Autodesk Inventor part; units mm, degrees
ref_plane "at507h_XY" through (0, 16.3576, 0) normal (0, 1, 0) x (1, 0, 0)
ref_plane "at507h_YZ" through (0, 16.3576, 0) normal (1, 0, 0) x (0, 0, -1)
ref_plane "at507h_ZX" through (0, 16.3576, 0) normal (0, 0, -1) x (0, 1, 0)
sketch "Sketch_1" plane through (0, 0, 0) normal (1, 0, 0) x (0, 1, 0)
  line L0 (12.8016, 6.5024) -> (9.7536, 6.5024)
  line L1 (9.7536, 6.5024) -> (9.7536, 5.4864)
  arc A0 (9.2456, 4.9784) -> (9.7536, 5.4864) centre (9.2456, 5.4864) ccw
  line L2 (9.2456, 4.9784) -> (2.54, 4.9784)
  line L3 (2.54, 4.9784) -> (2.54, -4.9784)
  line L4 (2.54, -4.9784) -> (9.2456, -4.9784)
  arc A1 (9.7536, -5.4864) -> (9.2456, -4.9784) centre (9.2456, -5.4864) ccw
  line L5 (9.7536, -5.4864) -> (9.7536, -6.5024)
  line L6 (9.7536, -6.5024) -> (12.8016, -6.5024)
  arc A2 (12.8016, -6.5024) -> (13.0556, -6.2484) centre (12.8016, -6.2484) ccw
  line L7 (13.0556, -6.2484) -> (13.0556, 6.2484)
  arc A3 (13.0556, 6.2484) -> (12.8016, 6.5024) centre (12.8016, 6.2484) ccw
extrude "Extrusion1" add sketch "Sketch_1" along normal mid plane 12.7
sketch "Sketch_2" plane through (0, 0, 0) normal (0, 1, 0) x (-1, 0, 0)
  line L0 (6.096, 6.2484) -> (-6.096, 6.2484)
  line L1 (-6.096, 6.2484) -> (-6.096, -6.2484)
  line L2 (-6.096, -6.2484) -> (6.096, -6.2484)
  line L3 (6.096, -6.2484) -> (6.096, 6.2484)
extrude "Extrusion2" cut sketch "Sketch_2" along normal blind 12.8016
sketch "Sketch_3" plane through (0, 0, 0) normal (0, 0, 1) x (1, 0, 0)
  line L0 (-6.35, 15.24) -> (-6.35, 12.8016)
  arc A0 (-6.096, 13.0556) -> (-6.35, 12.8016) centre (-6.096, 12.8016) ccw
  line L1 (-6.096, 13.0556) -> (6.096, 13.0556)
  arc A1 (6.35, 12.8016) -> (6.096, 13.0556) centre (6.096, 12.8016) ccw
  line L2 (6.35, 12.8016) -> (6.35, 15.24)
  line L3 (6.35, 15.24) -> (-6.35, 15.24)
extrude "Extrusion3" cut sketch "Sketch_3" along normal mid plane 25.6032
sketch "Sketch_4" plane through (0, 2.54, 0) normal (0, 1, 0) x (1, 0, 0)
  line L0 (-6.096, 5.4864) -> (-6.096, -5.4864)
  line L1 (-6.096, -5.4864) -> (-6.35, -5.4864)
  line L2 (-6.35, -5.4864) -> (-6.35, 5.4864)
  line L3 (-6.35, 5.4864) -> (-6.096, 5.4864)
  line L4 (-6.096, 5.4864) -> (-6.096, -5.4864)
revolve "Revolution1" add sketch "Sketch_4" angle 90 about axis through (-6.096, 2.54, -5.4864) along (0, 0, 1)
sketch "Sketch_5" plane through (0, 2.54, 0) normal (0, 1, 0) x (1, 0, 0)
  line L0 (6.096, -5.4864) -> (6.096, 5.4864)
  line L1 (6.096, 5.4864) -> (6.35, 5.4864)
  line L2 (6.35, 5.4864) -> (6.35, -5.4864)
  line L3 (6.35, -5.4864) -> (6.096, -5.4864)
  line L4 (6.096, -5.4864) -> (6.096, 5.4864)
revolve "Revolution2" add sketch "Sketch_5" angle 90 about axis through (6.096, 2.54, 5.4864) along (0, 0, -1)
sketch "Sketch_6" plane through (0, 2.54, 0) normal (0, 1, 0) x (1, 0, 0)
  line L0 (-6.096, 2.7305) -> (-6.096, -2.7305)
  line L1 (-6.096, -2.7305) -> (-5.715, -2.7305)
  arc A0 (-5.715, -2.7305) -> (-5.715, -1.9685) centre (-5.715, -2.3495) ccw
  line L2 (-5.715, -1.9685) -> (-5.715, 1.9685)
  arc A1 (-5.715, 1.9685) -> (-5.715, 2.7305) centre (-5.715, 2.3495) ccw
  line L3 (-5.715, 2.7305) -> (-6.096, 2.7305)
extrude "Extrusion4" add sketch "Sketch_6" against normal blind 0.254
sketch "Sketch_7" plane through (0, 2.54, 0) normal (0, 1, 0) x (1, 0, 0)
  arc A0 (5.715, 2.7305) -> (5.715, 1.9685) centre (5.715, 2.3495) ccw
  line L0 (5.715, 1.9685) -> (5.715, -1.9685)
  arc A1 (5.715, -1.9685) -> (5.715, -2.7305) centre (5.715, -2.3495) ccw
  line L1 (5.715, -2.7305) -> (6.096, -2.7305)
  line L2 (6.096, -2.7305) -> (6.096, 2.7305)
  line L3 (6.096, 2.7305) -> (5.715, 2.7305)
extrude "Extrusion5" add sketch "Sketch_7" against normal blind 0.254
sketch "Sketch_8" plane through (6.35, 0, 0) normal (1, 0, 0) x (0, 0, -1)
  line L0 (-7.1863, 0) -> (7.752, 0)
  line L1 (7.752, 0) -> (7.752, 3.302)
  line L2 (7.752, 3.302) -> (4.9784, 3.302)
  arc A0 (4.7244, 3.048) -> (4.9784, 3.302) centre (4.7244, 3.302) ccw
  line L3 (4.7244, 3.048) -> (2.9845, 3.048)
  arc A1 (2.9845, 3.048) -> (2.7305, 2.794) centre (2.9845, 2.794) ccw
  line L4 (2.7305, 2.794) -> (2.7305, 2.286)
  line L5 (2.7305, 2.286) -> (1.9685, 2.286)
  line L6 (1.9685, 2.286) -> (1.9685, 2.794)
  arc A2 (1.9685, 2.794) -> (1.7145, 3.048) centre (1.7145, 2.794) ccw
  line L7 (1.7145, 3.048) -> (-1.7145, 3.048)
  arc A3 (-1.7145, 3.048) -> (-1.9685, 2.794) centre (-1.7145, 2.794) ccw
  line L8 (-1.9685, 2.794) -> (-1.9685, 2.286)
  line L9 (-1.9685, 2.286) -> (-2.7305, 2.286)
  line L10 (-2.7305, 2.286) -> (-2.7305, 2.794)
  arc A4 (-2.7305, 2.794) -> (-2.9845, 3.048) centre (-2.9845, 2.794) ccw
  line L11 (-2.9845, 3.048) -> (-4.7244, 3.048)
  arc A5 (-4.9784, 3.302) -> (-4.7244, 3.048) centre (-4.7244, 3.302) ccw
  line L12 (-4.9784, 3.302) -> (-7.1863, 3.302)
  line L13 (-7.1863, 3.302) -> (-7.1863, 0)
extrude "Extrusion6" cut sketch "Sketch_8" against normal blind 25.4
sketch "Sketch_17" plane through (0, 0, 0) normal (0, 0, 1) x (1, 0, 0)
  line L0 (0, 13.0556) -> (0, 21.9456)
  line L1 (0, 21.9456) -> (3.175, 21.9456)
  line L2 (3.175, 21.9456) -> (3.175, 13.9446)
  line L3 (3.175, 13.9446) -> (3.683, 13.9446)
  line L4 (3.683, 13.9446) -> (3.683, 13.0556)
  line L5 (3.683, 13.0556) -> (0, 13.0556)
  line L6 (0, 13.0556) -> (0, 21.9456)
revolve "Revolution3" add sketch "Sketch_17" angle 360 about axis through (0, 13.0556, 0) along (0, -1, 0)
thread "Thread1"
sketch "Sketch_19" plane through (0, 0, 0) normal (0, 0, 1) x (1, 0, 0)
  line L0 (0, 20.6756) -> (0, 21.9456)
  line L1 (0, 21.9456) -> (2.159, 21.9456)
  line L2 (2.159, 21.9456) -> (2.159, 20.6756)
  line L3 (2.159, 20.6756) -> (0, 20.6756)
  line L4 (0, 20.6756) -> (0, 21.9456)
revolve "Revolution4" cut sketch "Sketch_19" angle 360 about axis through (0, 20.6756, 0) along (0, -1, 0)
sketch "Sketch_35" plane through (0, 14.7066, 0) normal (0, 1, 0) x (1, 0, 0)
  line L0 (-0.254, -3.175) -> (0.254, -3.175)
  line L1 (0.254, -3.175) -> (0.254, -2.6518)
  line L2 (0.254, -2.6518) -> (-0.254, -2.6518)
  line L3 (-0.254, -2.6518) -> (-0.254, -3.175)
extrude "Extrusion7" cut sketch "Sketch_35" along normal blind 20.32
ref_plane "at507h_XY" through (0, 16.3576, 0) normal (0, 1, 0) x (1, 0, 0)
ref_plane "at507h_YZ" through (0, 16.3576, 0) normal (1, 0, 0) x (0, 0, -1)
ref_plane "at507h_ZX" through (0, 16.3576, 0) normal (0, 0, -1) x (0, 1, 0)
ref_plane "at507h_dual_XY" through (-2.4003, 16.3576, 0) normal (0, 1, 0) x (1, 0, 0)
ref_plane "at507h_dual_YZ" through (-2.4003, 16.3576, 0) normal (1, 0, 0) x (0, 0, -1)
ref_plane "at507h_dual_ZX" through (-2.4003, 16.3576, 0) normal (0, 0, -1) x (0, 1, 0)
ref_plane "at509_XY" through (0, 15.7099, 0) normal (0, 1, 0) x (1, 0, 0)
ref_plane "at509_YZ" through (0, 15.7099, 0) normal (1, 0, 0) x (0, 0, -1)
ref_plane "at509_ZX" through (0, 15.7099, 0) normal (0, 0, -1) x (0, 1, 0)
ref_plane "at509_dual_XY" through (-2.4003, 15.7099, 0) normal (0, 1, 0) x (1, 0, 0)
ref_plane "at509_dual_YZ" through (-2.4003, 15.7099, 0) normal (1, 0, 0) x (0, 0, -1)
ref_plane "at509_dual_ZX" through (-2.4003, 15.7099, 0) normal (0, 0, -1) x (0, 1, 0)
ref_plane "at513h_XY" through (0, 14.7066, 0) normal (0, 1, 0) x (1, 0, 0)
ref_plane "at513h_YZ" through (0, 14.7066, 0) normal (1, 0, 0) x (0, 0, -1)
ref_plane "at513h_ZX" through (0, 14.7066, 0) normal (0, 0, -1) x (0, 1, 0)
ref_plane "at513h_dual_XY" through (-2.4003, 14.7066, 0) normal (0, 1, 0) x (1, 0, 0)
ref_plane "at513h_dual_YZ" through (-2.4003, 14.7066, 0) normal (1, 0, 0) x (0, 0, -1)
ref_plane "at513h_dual_ZX" through (-2.4003, 14.7066, 0) normal (0, 0, -1) x (0, 1, 0)
ref_plane "body_c_to_bracket_XY" through (0, 13.0556, 0) normal (0, -1, 0) x (1, 0, 0)
ref_plane "body_c_to_bracket_YZ" through (0, 13.0556, 0) normal (1, 0, 0) x (0, 0, 1)
ref_plane "body_c_to_bracket_ZX" through (0, 13.0556, 0) normal (0, 0, 1) x (0, -1, 0)
ref_plane "body_cover_to_body_XY" through (0, 12.8016, 0) normal (0, 1, 0) x (1, 0, 0)
ref_plane "body_cover_to_body_YZ" through (0, 12.8016, 0) normal (1, 0, 0) x (0, 0, -1)
ref_plane "body_cover_to_body_ZX" through (0, 12.8016, 0) normal (0, 0, -1) x (0, 1, 0)
ref_plane "body_cover_to_toggle_XY" through (0, 18.1356, 0) normal (0, 1, 0) x (1, 0, 0)
ref_plane "body_cover_to_toggle_YZ" through (0, 18.1356, 0) normal (1, 0, 0) x (0, 0, -1)
ref_plane "body_cover_to_toggle_ZX" through (0, 18.1356, 0) normal (0, 0, -1) x (0, 1, 0)
ref_plane "body_cover_to_toggle2_XY" through (-2.4003, 18.1356, 0) normal (0, 1, 0) x (1, 0, 0)
ref_plane "body_cover_to_toggle2_YZ" through (-2.4003, 18.1356, 0) normal (1, 0, 0) x (0, 0, -1)
ref_plane "body_cover_to_toggle2_ZX" through (-2.4003, 18.1356, 0) normal (0, 0, -1) x (0, 1, 0)
ref_plane "st513h_2_XY" through (0, 17.5006, 0) normal (0, 1, 0) x (1, 0, 0)
ref_plane "st513h_2_YZ" through (0, 17.5006, 0) normal (1, 0, 0) x (0, 0, -1)
ref_plane "st513h_2_ZX" through (0, 17.5006, 0) normal (0, 0, -1) x (0, 1, 0)
ref_plane "st513h_2_dual_XY" through (-2.4003, 17.5006, 0) normal (0, 1, 0) x (1, 0, 0)
ref_plane "st513h_2_dual_YZ" through (-2.4003, 17.5006, 0) normal (1, 0, 0) x (0, 0, -1)
ref_plane "st513h_2_dual_ZX" through (-2.4003, 17.5006, 0) normal (0, 0, -1) x (0, 1, 0)
properties part number "M211LW01-body-cover"
Here's how the part is built. I have some questions about the finished solid (model axes, mm). A direction names the side the tool comes from. Round coordinates to 2 decimals unless told otherwise and drop trailing zeros. Loops run counter-clockwise (first coordinate to the right, second up) from the corner with the lowest first, then second, coordinate; pieces in that order, holes last. Notation, with made-up numbers: (87.5, 76.5) -> (127.5, 76.5) arc R15 ccw to (127.5, 82.5) -> close; hole circle Ø5 at (7, 43). An arc over 180 degrees is marked (long way). Answer as CSV lines item,"result". Start each with the question number.
1. Imagine slicing it at A-A on y = 12.5. Write out the boundary of the cut face in (x, z).
2. If we mould it in two halves opening along Z, with no side actions, what happens to faces 5 (the face through (0, 11, 6.502)), 6 (the face through (6.35, 9, 0)), 7 (the face through (1.699, 13.494, -3.267)), 8 (the face through (-6.096, 9, 0))? For each: pulls with the +Z half, pulls with the -Z half, needs draft (parallel to the pull), parting line crosses it, or undercut.
3. I'm going to push flat-ended pins straight in: P1, Ø0.6, axis at x = 6, y = 2.5, coming from the +Z side; P2, Ø1, axis at y = 14.5, z = -5, coming from the +X side; P3, Ø3, axis at x = -1.5, z = 4.5, coming from the +Y side. Where does each tip first touch, or does it pass through?
4. Imagine slicing it at B-B on x = -4.75. Write out the boundary of the cut face in (y, z), plus the area to 3 significant figures.
5. For faces 1 (the face through (6.096, 8, 0)), 2 (the face through (0, 11, 6.248)), 3 (the face through (-6.35, 9, 0)), 4 (the face through (-0.28, 21.3, 2.14)), which set-ups out of +Z, -Z, +X, -X, +Y, -Y let a thin tool reach every point of the face, with its end or its side?
6. I need wall thicknesses on probe 1 along Z at (x, y) = (0, 21) (3 decimals); probe 2 along Y at (x, z) = (-5.5, 2.25); probe 3 along X at (y, z) = (10.25, -0.25). Which ranges of each line are inside material? Lowest first, please. Write a range as from..to.
7. Imagine slicing it at C-C on y = 4.25. Write out the boundary of the cut face in (x, z), plus the area to 3 significant figures.
8. Imagine slicing it at D-D on z = -4. Write out the boundary of the cut face in (x, y).
Solution:
1,outline,"(-6.35, -6.5) -> (6.35, -6.5) -> (6.35, 6.5) -> (-6.35, 6.5) -> close; hole (-6.1, -6.25) -> (6.1, -6.25) -> (6.1, 6.25) -> (-6.1, 6.25) -> close"
2,face 5,"pulls with the +Z half"
2,face 6,"needs draft"
2,face 7,"parting line crosses it"
2,face 8,"undercut"
3,P1,"z = 2.73"
3,P2,"through"
3,P3,"y = 13.94"
4,outline,"(9.75, -6.5) -> (12.8, -6.5) arc R0.25 ccw to (13.06, -6.25) -> (13.06, 6.25) arc R0.25 ccw to (12.8, 6.5) -> (9.75, 6.5) -> (9.75, 6.25) -> (12.8, 6.25) -> (12.8, -6.25) -> (9.75, -6.25) -> close"
4,area,"4.82 mm²"
5,face 1,"none"
5,face 2,"-Y"
5,face 3,"+Z, -Z, -X, +Y, -Y"
5,face 4,"+Y"
6,probe 1,"-3.175..-2.159, 2.159..2.652"
6,probe 2,"2.29..2.54, 12.8..13.06"
6,probe 3,"-6.35..-6.1, 6.1..6.35"
7,outline,"(-6.35, -4.98) -> (-6.1, -4.98) -> (-6.1, 4.98) -> (-6.35, 4.98) -> close; (6.1, -4.98) -> (6.35, -4.98) -> (6.35, 4.98) -> (6.1, 4.98) -> close"
7,area,"5.06 mm²"
8,outline,"(-6.35, 3.05) -> (-6.1, 3.05) -> (-6.1, 12.8) -> (6.1, 12.8) -> (6.1, 3.05) -> (6.35, 3.05) -> (6.35, 12.8) arc R0.25 ccw to (6.1, 13.06) -> (-6.1, 13.06) arc R0.25 ccw to (-6.35, 12.8) -> close"
